Check sheet for the modelled part. Datum: model origin and axes. Units: mm. A direction names the side the tool comes from. Give positions to 0.01 mm unless a question says otherwise; leave off trailing zeros. Write each loop counter-clockwise with the first axis right and the second up, starting at its lowest first coordinate (ties: lowest second). Pieces come first, ordered by that corner, then holes. Notation, with made-up numbers: (84, 76.5) -> (95, 76.5) arc R8 ccw to (95, 83.5) -> close; hole circle Ø5 at (12.5, -16.5). An arc over 180 degrees is marked (long way). Use a Markdown table: item, result. Add a question column.
1. Cross-section at B-B (x = 39). Enter the section's corners in (y, z).
2. Cross-section at A-A (z = 20). Enter the section's corners in (x, y).
3. Release check for a two-part mould opening along X. For faces 6 (the cylindrical face through (-12.858, 7.395, 22.727)), 7 (the cylindrical face through (-57.616, 105.162, 19.72)), 8 (the flat face through (43, 160, 20)) record: released by +X, released by -X, zero draft, split by the parting line, or undercut.
4. Set-up check for faces 1 (the flat face through (35, 170, 20)), 2 (the flat face through (-11, 15, 23)), 3 (the flat face through (0, 8, 20)), 4 (the flat face through (-25, 10, 20)), 5 (the cylindrical face through (45.14, 170.79, 5.63)): record each of +Z, -Z, +X, -X, +Y, -Y from which the full face is reachable in a straight line by a thin tool's end or side.
5. Cross-section at C-C (x = -20.5). Enter the section's corners in (y, z), then the cut area to 3 significant figures.
6. Scan lines: probe 1 along Y at (x, z) = (47, 34.75); probe 2 along Z at (x, y) = (-12.5, 11.5); probe 3 along Z at (x, y) = (-12.5, 20.5). Record each from-to range of solid material in increasing order. Write a range as [from, to].
7. Cross-section at D-D (x = 7). Enter the section's corners in (y, z), then the cut area to 3 significant figures.
8. Gauge pin test, flat ends, axial feed: P1, Ø6, axis at x = 47, z = 28.5, coming from the -Y side; P2, Ø23.5, axis at y = 10, z = 21, coming from the -X side; P3, Ø1, axis at y = 38.5, z = 8.5, coming from the -X side. Record the tip position at first contact, or that the pin passes through.
from build123d import *

# Parameters (mm, degrees)
BOSS_EXTRUDE1_DEPTH = 40
SKETCH2_R           = 9.5
CUT_EXTRUDE1_DEPTH  = 186
SKETCH3_R           = 2.75
CUT_EXTRUDE2_DEPTH  = 40
CUT_EXTRUDE3_START  = -15
SKETCH4_R           = 5.5
CUT_EXTRUDE3_DEPTH  = 29
SKETCH5_R           = 1.75
CUT_EXTRUDE4_DEPTH  = 31


with BuildPart() as part:
    # Sketch1 → Boss-Extrude1 (new body)
    with BuildSketch(Plane.XY):
        with BuildLine():
            ThreePointArc((0, 180), (-47.896390796, 97.5), (0, 15))
            Line((0, 15), (0, 0))
            Line((0, 0), (-25, 0))
            Line((-25, 0), (-25, 21.171305921))
            ThreePointArc((-25, 21.171305921), (-57.511689732, 106.47993478), (-10.937324628, 185))
            Line((-10.937324628, 185), (55, 185))
            Line((55, 185), (55, 160))
            Line((55, 160), (35, 160))
            Line((35, 160), (35, 180))
            Line((35, 180), (0, 180))
        make_face()
    extrude(amount=BOSS_EXTRUDE1_DEPTH)

    # Sketch2 → Cut-Extrude1 (cut, through all)
    with BuildSketch(Plane(origin=(0, 185, 0), x_dir=(1, 0, 0), z_dir=(0, 1, 0))):
        with Locations((55, -20)):
            Circle(SKETCH2_R)
    extrude(amount=-CUT_EXTRUDE1_DEPTH, mode=Mode.SUBTRACT)

    # Sketch3 → Cut-Extrude2 (cut)
    with BuildSketch(Plane.XZ):
        with Locations((-12.5, 20)):
            Circle(SKETCH3_R)
    extrude(amount=-CUT_EXTRUDE2_DEPTH, mode=Mode.SUBTRACT)

    # Sketch4 → Cut-Extrude3 (cut)
    with BuildSketch(Plane.XZ.offset(CUT_EXTRUDE3_START)):
        with Locations((-12.5, 20)):
            Circle(SKETCH4_R)
    extrude(amount=-CUT_EXTRUDE3_DEPTH, mode=Mode.SUBTRACT)

    # Sketch5 → Cut-Extrude4 (cut)
    with BuildSketch(Plane(origin=(55, 0, 0), x_dir=(0, 0, -1), z_dir=(1, 0, 0))):
        with Locations((-5.25, 172.5)):
            Circle(SKETCH5_R)
        with Locations((-34.75, 172.5)):
            Circle(SKETCH5_R)
    extrude(amount=-CUT_EXTRUDE4_DEPTH, mode=Mode.SUBTRACT)


solid = part.part
Worked answers:
| question | item | result |
|---|---|---|
| 1 | outline | (160, 0) -> (185, 0) -> (185, 40) -> (160, 40) -> close; hole circle Ø3.5 at (172.5, 5.25); hole circle Ø3.5 at (172.5, 34.75) |
| 2 | outline | (-25, 0) -> (-15.25, 0) -> (-15.25, 15) -> (-18, 15) -> (-18, 28.32) arc R95 cw to (0, 180) -> (35, 180) -> (35, 160) -> (45.5, 160) -> (45.5, 185) -> (-10.94, 185) arc R105 ccw to (-25, 21.17) -> close; (-9.75, 0) -> (0, 0) -> (0, 15) arc R95 cw to (-7, 19.41) -> (-7, 15) -> (-9.75, 15) -> close |
| 3 | face 6 | undercut |
| 3 | face 7 | released by -X |
| 3 | face 8 | zero draft |
| 4 | face 1 | +Z, -Z, -Y |
| 4 | face 2 | none |
| 4 | face 3 | +Z, -Z, +X, -Y |
| 4 | face 4 | +Z, -Z, -X, -Y |
| 4 | face 5 | +X |
| 5 | outline | (0, 0) -> (30.76, 0) -> (30.76, 40) -> (0, 40) -> close; (164.24, 0) -> (177.84, 0) -> (177.84, 40) -> (164.24, 40) -> close |
| 5 | area | 1,770 mm² |
| 6 | probe 1 | y = [160, 170.75], [174.25, 185] |
| 6 | probe 2 | z = [0, 17.25], [22.75, 40] |
| 6 | probe 3 | z = [0, 14.5], [25.5, 40] |
| 7 | outline | (180, 0) -> (185, 0) -> (185, 40) -> (180, 40) -> close |
| 7 | area | 200 mm² |
| 8 | P1 | stops at y = 160 |
| 8 | P2 | stops at x = -25.61 |
| 8 | P3 | stops at x = -40.09 |
